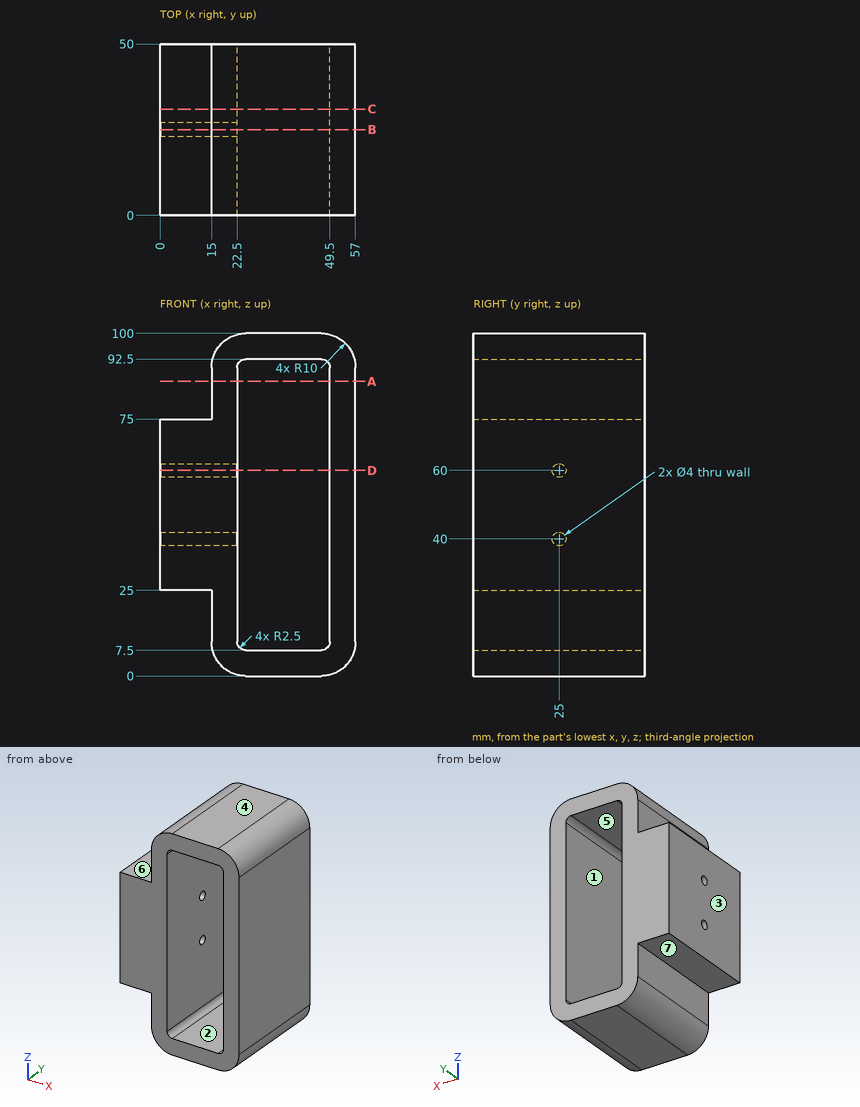
Design review of the part shown in the three views and the two pictorial views. Dimensions are in mm from the part's minimum x, y and z. A direction names the side the tool comes from. Coordinates: 2 decimals unless noted, no trailing zeros. Loops run counter-clockwise (first coordinate to the right, second up) from the corner with the lowest first, then second, coordinate; pieces in that order, holes last. Notation, with made-up numbers: M -17,17.25 L 4,17.25 A13 cw 4,31.25 Z; hole C -10.75,-26 d7. An arc over 180 degrees is marked long. Put each result on its own line as item: value. Start each with the question number.
Q1. Add section A-A (z = 86). Write out the cut boundary in (x, y).
Q2. Wall thickness on line 1 (X direction, y = 10, z = 51.5); line 2 (Y direction, x = 16.25, z = 60); line 3 (Z direction, x = 29, y = 2.5): over which ranges is each line inside the solid? List them lowest first.
Q3. Clearance check with flat-ended pins moving along their axes: pin 1 (5 mm diameter, centred on x = 10.5, y = 20.5, fed in from -Z); pin 2 (7.5 mm diameter, centred on y = 30.5, z = 19, fed in from -X); pin 3 (5 mm diameter, centred on x = 16.5, y = 21, fed in from -Z). State where each tip first meets the part, or that it passes through.
Q4. For the marked faces 5, 6 and 7, list the 3-axis set-ups (+Z, -Z, +X, -X, +Y, -Y) from which the entire face can be reached by the end or side of a thin tool; tool diameter is ignored.
Q5. Add section B-B (y = 25). Write out the cut boundary in (x, z), and give its area (3 significant figures).
Q6. The part is to be moulded in two halves that separate along Z. For the marked faces 1, 2, 3 and 4, say which applies: +Z half, -Z half, draft (parallel to the pull), parting line (faces both ways), or undercut.
Q7. Add section C-C (y = 31). Write out the cut boundary in (x, z), and give its area (3 significant figures).
Q8. Add section D-D (z = 60). Write out the cut boundary in (x, y).
Answers:
1. outline: M 15,0 L 22.5,0 L 22.5,50 L 15,50 Z; M 49.5,0 L 57,0 L 57,50 L 49.5,50 Z
2. line 1: x = 0 to 22.5, 49.5 to 57
2. line 2: y = 0 to 23, 27 to 50
2. line 3: z = 0 to 7.5, 92.5 to 100
3. pin 1: stops at z = 25
3. pin 2: stops at x = 15
3. pin 3: stops at z = 2
4. face 5: +Y, -Y
4. face 6: +Z, -X, +Y, -Y
4. face 7: -Z, -X, +Y, -Y
5. outline: M 0,25 L 15,25 L 15,10 A10 ccw 25,0 L 47,0 A10 ccw 57,10 L 57,90 A10 ccw 47,100 L 25,100 A10 ccw 15,90 L 15,75 L 0,75 L 0,62 L 22.5,62 L 22.5,90 A2.5 cw 25,92.5 L 47,92.5 A2.5 cw 49.5,90 L 49.5,10 A2.5 cw 47,7.5 L 25,7.5 A2.5 cw 22.5,10 L 22.5,38 L 0,38 Z; M 0,42 L 22.5,42 L 22.5,58 L 0,58 Z
5. area: 2,390 mm^2
6. face 1: undercut
6. face 2: undercut
6. face 3: draft
6. face 4: +Z half
7. outline: M 0,25 L 15,25 L 15,10 A10 ccw 25,0 L 47,0 A10 ccw 57,10 L 57,90 A10 ccw 47,100 L 25,100 A10 ccw 15,90 L 15,75 L 0,75 Z; hole M 22.5,10 A2.5 ccw 25,7.5 L 47,7.5 A2.5 ccw 49.5,10 L 49.5,90 A2.5 ccw 47,92.5 L 25,92.5 A2.5 ccw 22.5,90 Z
7. area: 2,570 mm^2
8. outline: M 0,0 L 22.5,0 L 22.5,23 L 0,23 Z; M 0,27 L 22.5,27 L 22.5,50 L 0,50 Z; M 49.5,0 L 57,0 L 57,50 L 49.5,50 Z
